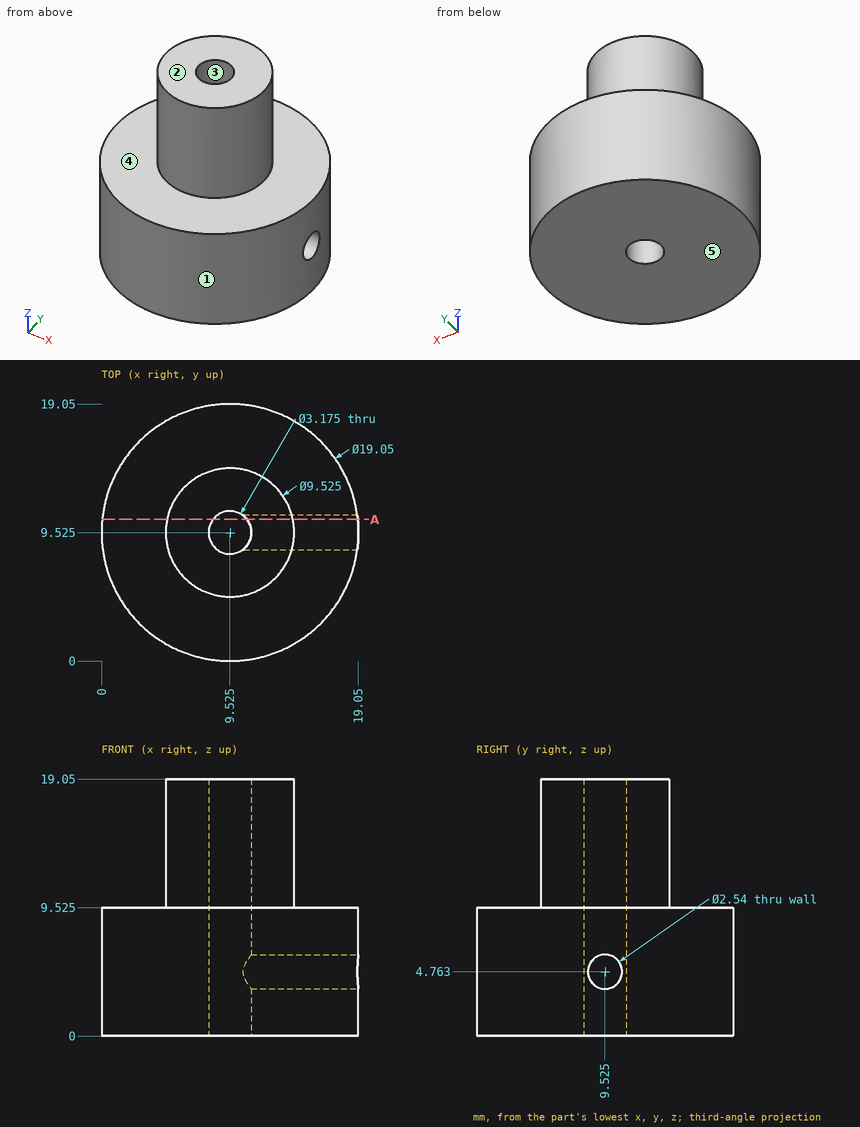
Check sheet for the drawn part. Datum: minimum x, y, z corner. Units: mm. A direction names the side the tool comes from. Round coordinates to 2 decimals unless told otherwise and drop trailing zeros. Write each question's results on one line, items separated by ' | '. Start each with the question number.
1. Go/stop test with flat-tipped pins: P1, Ø3, axis at x = 6, z = 7, coming from the +Y side; P2, Ø4, axis at y = 9.53, z = 4.76, coming from the +X side; P3, Ø1, axis at y = 3, z = 16.5, coming from the +X side; P4, Ø10, axis at x = 8, z = 15, coming from the -Y side. Record where each tip stops, or that it passes through.
2. Draft check along X on the marked faces 1, 2 and 3. Enter one of: pulls with the +X half, pulls with the -X half, needs draft (parallel to the pull), parting line crosses it, or undercut.
3. Material ranges on L1, parallel to Z at x = 4, y = 14 (1 decimal); L2, parallel to X at y = 10.5, z = 16 (1 decimal); L3, parallel to Y at x = 9.75, z = 5, recorded low to high. Write a range as from..to.
4. Set-up check for the marked faces 4 and 5: record each of +Z, -Z, +X, -X, +Y, -Y from which the full face is reachable in a straight line by a thin tool's end or side.
5. Cross-section at A-A on y = 10.5. Give the number of separate pieces and of enclosed holes in the cut face, plus the area to 3 significant figures.
Resolved:
1) P1: y = 18.83 | P2: x = 19.05 | P3: through | P4: y = 4.76
2) face 1: parting line crosses it | face 2: needs draft | face 3: undercut
3) L1: 0..9.5 | L2: 4.9..8.3, 10.8..14.2 | L3: 0..7.95, 11.1..19.05
4) face 4: +Z | face 5: -Z, +X, -X, +Y, -Y
5) separate pieces: 3 | enclosed holes: 0 | area: 208 mm2
